Design review of the part built by this model. Coordinates are the model's own, in mm. A direction names the side the tool comes from. Round coordinates to 2 decimals unless told otherwise and drop trailing zeros. Order: outer loops, then holes, each group sorted by start corner. A loop starts at its lowest first (then second) coordinate and runs counter-clockwise, first axis right, second up. Notation, with made-up numbers: M -13,-15.5 L -9,-15.5 A30 ccw -9,7.5 Z; hole C 32.5,41 d8. An arc over 180 degrees is marked long. Write each question's results on one line, items separated by ' | '. Start each with the question number.
Item 1: Clearance check with flat-ended pins moving along their axes: pin 1 (1 mm diameter, centred on x = 29, z = -67.5, fed in from -Y); pin 2 (7 mm diameter, centred on x = 40, z = -69, fed in from -Y); pin 3 (8 mm diameter, centred on y = -22, z = -56.5, fed in from +X); pin 4 (8 mm diameter, centred on y = -18, z = -38.5, fed in from -X). State where each tip first meets the part, or that it passes through.
Item 2: Take a section at C-C, the plane z = -17.5. Write out the cut boundary in (x, y).
Item 3: Take a section at B-B, the plane y = -19. Write out the cut boundary in (x, z).
Item 4: Wall thickness on line 1 (X direction, y = -22, z = -69); line 2 (Z direction, x = 40, y = -20.75); line 3 (Y direction, x = 33, z = -64.5): over which ranges is each line inside the solid? List them lowest first. Write a range as [from, to].
Item 5: Machinability: for faces 4 (the flat face through (40, -25, -39)), 5 (the flat face through (55, -20, -39)), 6 (the flat face through (41, -30, 10)), 7 (the flat face through (40, -15, -39)), which of the approach directions +Z, -Z, +X, -X, +Y, -Y give a long, thin tool a straight path to every point of the face, cutting with its end or side? Answer none if there is none.
Item 6: The part is to be moulded in two halves that separate along X. For faces 1 (the cylindrical face through (36.034, -20.07, -69.521)), 2 (the flat face through (39, -19, 20)), 3 (the flat face through (25, -20, -40)), say which applies: +X half, -X half, draft (parallel to the pull), parting line (faces both ways), or undercut.
Item 7: Take a section at A-A, the plane z = -69. Write out the cut boundary in (x, y).
Autodesk Inventor part; units mm, degrees
ref_plane "YZ Plane" through (0, 0, 0) normal (1, 0, 0) x (0, 1, 0)
ref_plane "XZ Plane" through (0, 0, 0) normal (0, 1, 0) x (-1, 0, 0)
ref_plane "XY Plane" through (0, 0, 0) normal (0, 0, 1) x (1, 0, 0)
sketch "Sketch3" plane through (0, 0, 0) normal (0, 0, 1) x (1, 0, 0)
  line L0 (0, 0) -> (80, 0)
  line L1 (80, 0) -> (80, -30)
  line L2 (80, -30) -> (0, -30)
  line L3 (0, -30) -> (0, 0)
  line L4 (0, 0) -> (14.7083, -12.3417) construction
  line L5 (14.7083, -12.3417) -> (40, -15) construction
  line L6 (40, -15) -> (65.2917, -12.3417) construction
  line L7 (65.2917, -12.3417) -> (80, 0) construction
  spline S0 degree 4 poles (0, 0) (14.7083, -12.3417) (40, -15) (65.2917, -12.3417) (80, 0) knots 1 1 1 1 1 2 2 2 2 2
  point P0 (52.6458, -13.6709)
  dimension "d13" = 80
  dimension "d14" = 30
  dimension "d15" = 15
  dimension "d16" = 40
  dimension "d17" = 50
  dimension "d18" = 50
  dimension "d19" = 6
  dimension "d21" = 6
extrude "Extrusion1" add sketch "Sketch3" along normal blind 20 contours S0 L1 L2 L3
sketch "Sketch4" plane through (0, 0, 0) normal (0, 0, -1) x (-1, 0, 0)
  line L0 (-25, -25) -> (-55, -25)
  line L1 (-55, -25) -> (-55, -15)
  line L2 (-55, -15) -> (-25, -15)
  line L3 (-25, -15) -> (-25, -25)
  line L4 (-40, -25) -> (-40, -15) construction
  line L5 (-80, -30) -> (-80, 0)
  line L6 (0, -30) -> (-80, -30)
  point P0 (0, 0)
  dimension "d24" = 30
  dimension "d25" = 40
  dimension "d26" = 5
  dimension "d27" = 10
extrude "Extrusion2" add sketch "Sketch4" along normal blind 80
sketch "Sketch7" plane through (25, -15, 0) normal (0, 1, 0) x (1, 0, 0)
  line L0 (0, 55) -> (20, 55)
  line L1 (20, 55) -> (20, 75)
  line L2 (20, 75) -> (0, 75)
  line L3 (0, 75) -> (0, 55)
  line L4 (30, 0) -> (0, 0)
  line L5 (30, 0) -> (30, 80)
  line L6 (0, 80) -> (30, 80)
  line L7 (0, 0) -> (0, 80)
  circle A0 centre (10, 65) radius 4
  line L8 (0, 55) -> (0, 55)
  line L9 (0, 0) -> (0, 80)
  line L10 (20, 55) -> (30, 55)
  point P0 (-25, 0)
  point P1 (20, 65)
  point P2 (10, 75)
  point P3 (0, 35)
  dimension "d40" = 10
  dimension "d42" = 20
  dimension "d43" = 20
  dimension "d44" = 8
  dimension "d51" = 15
extrude "Extrusion4" add sketch "Sketch7" along normal blind 10 contours L3 L2 L1 L0 | L1 L2 L7 L6 L5 L10 | A0
sketch "Sketch9" plane through (0, 0, -80) normal (0, 0, -1) x (-1, 0, 0)
  line L0 (-55, -25) -> (-55, -5)
  line L1 (-55, -25) -> (-25, -25)
  line L2 (-25, -25) -> (-25, -5)
  line L3 (-55, -5) -> (-25, -5)
  point P0 (0, 0)
extrude "Extrusion7" cut sketch "Sketch9" against normal blind 19
sketch "Sketch10" plane through (0, 0, -61) normal (0, 0, -1) x (-1, 0, 0)
  line L0 (-40, -5) -> (-40, -25) construction
  line L1 (-25, -5) -> (-55, -5)
  line L2 (-25, -25) -> (-55, -25)
  line L3 (-55, -5) -> (-25, -5)
  line L4 (-25, -5) -> (-25, -25)
  line L5 (-25, -25) -> (-55, -25)
  line L6 (-55, -25) -> (-55, -5)
  line L7 (-55, -25) -> (-55, -5)
  line L8 (-25, -5) -> (-25, -25)
  line L9 (-55, -15) -> (-25, -15)
  line L10 (-25, -15) -> (-25, -25)
  line L11 (-25, -25) -> (-55, -25)
  line L12 (-55, -25) -> (-55, -15)
  point P0 (0, 0)
  dimension "d81" = 10
extrude "Extrusion10" add sketch "Sketch10" along normal blind 18
sketch "Sketch12" plane through (25, -5, 0) normal (0, 1, 0) x (1, 0, 0)
  line L0 (0, 79) -> (0, 55)
  line L1 (0, 55) -> (30, 55)
  line L2 (30, 55) -> (30, 79)
  line L3 (0, 79) -> (30, 79)
  line L4 (0, 0) -> (0, 79)
  line L5 (30, 0) -> (30, 79)
  line L6 (0, 79) -> (30, 79)
  line L7 (30, 79) -> (30, 64)
  line L8 (30, 64) -> (0, 64)
  line L9 (0, 64) -> (0, 79)
  point P0 (-25, 0)
  point P1 (0, 64)
  dimension "d84" = 15
extrude "Extrusion11" cut sketch "Sketch12" against normal blind 15 contours L3 L2 L8 L0
sketch "Sketch13" plane through (25, -20, 0) normal (0, 1, 0) x (1, 0, 0)
  line L0 (30, 79) -> (30, 64)
  line L1 (0, 79) -> (30, 79)
  line L2 (0, 64) -> (0, 79)
  line L3 (30, 64) -> (0, 64)
  circle A0 centre (7, 71.5) radius 4
  circle A1 centre (23, 71.5) radius 4
  circle A2 centre (7, 71.5) radius 6
  circle A3 centre (23, 71.5) radius 6
  point P0 (-25, 0)
  point P1 (0, 71.5)
  dimension "d87" = 8
  dimension "d88" = 8
  dimension "d89" = 7.5
  dimension "d90" = 7.5
  dimension "d91" = 7
  dimension "d92" = 7
  dimension "d93" = 2
  dimension "d94" = 2
extrude "Extrusion14" add sketch "Sketch13" along normal blind 15 contours L0 L3 L2 L1 | A0 | A1 | A2 | A3
sketch "Sketch14" plane through (25, -15, 0) normal (0, 1, 0) x (1, 0, 0)
  line L0 (30, 0) -> (30, 79)
  line L1 (30, 55) -> (0, 55)
  line L2 (0, 55) -> (0, 39)
  line L3 (0, 39) -> (30, 39)
  line L4 (30, 39) -> (30, 55)
  line L5 (30, 55) -> (0, 55)
  point P0 (-25, 0)
  point P1 (30, 39)
  dimension "d101" = 30
  dimension "d102" = 16
extrude "Extrusion15" add sketch "Sketch14" along normal up to surface (10 mm away)
sketch "Sketch15" plane through (25, -5, 0) normal (0, 1, 0) x (1, 0, 0)
  line L0 (30, 79) -> (0, 79)
  line L1 (0, 79) -> (0, 39)
  point P0 (-25, 0)
  point P1 (15, 69)
  dimension "d105" = 10
  dimension "d106" = 15
hole "Hole1" at (40, -5, -69) direction (0, -1, 0) diameter 8 depth 20
sketch "Sketch16" plane through (25, -5, 0) normal (0, 1, 0) x (1, 0, 0)
  circle A0 centre (15, 69) radius 4
  line L0 (0, 79) -> (0, 39)
  line L1 (30, 39) -> (0, 39)
  line L2 (30, 79) -> (30, 39)
  line L3 (30, 79) -> (0, 79)
  point P0 (-25, 0)
extrude "Extrusion16" cut sketch "Sketch16" against normal up to surface (10 mm away)
fillet "Fillet1" radius 2 2 edges at (80, 0, 10) (0, 0, 10)
thread "Thread1"
properties part number "Part 1 menton" material "ABS Plastic"
Results list:
1) pin 1: y = -25 | pin 2: through | pin 3: x = 55 | pin 4: x = 25
2) outline: M 25,-25 L 55,-25 L 55,-15 L 25,-15 Z
3) outline: M 0,0 L 25,0 L 25,-79 L 55,-79 L 55,0 L 80,0 L 80,20 L 0,20 Z; hole C 40,-69 d8
4) line 1: [25, 36], [44, 55] | line 2: [-79, -73], [-65, 20] | line 3: [-25, -15]
5) face 4: -Z, +X, -X, -Y | face 5: -Z, +X, +Y, -Y | face 6: +Z, -Z, +X, -X, -Y | face 7: -Z, +X, -X, +Y
6) face 1: undercut | face 2: draft | face 3: -X half
7) outline: M 25,-25 L 36,-25 L 36,-15 L 25,-15 Z; M 44,-25 L 55,-25 L 55,-15 L 44,-15 Z
